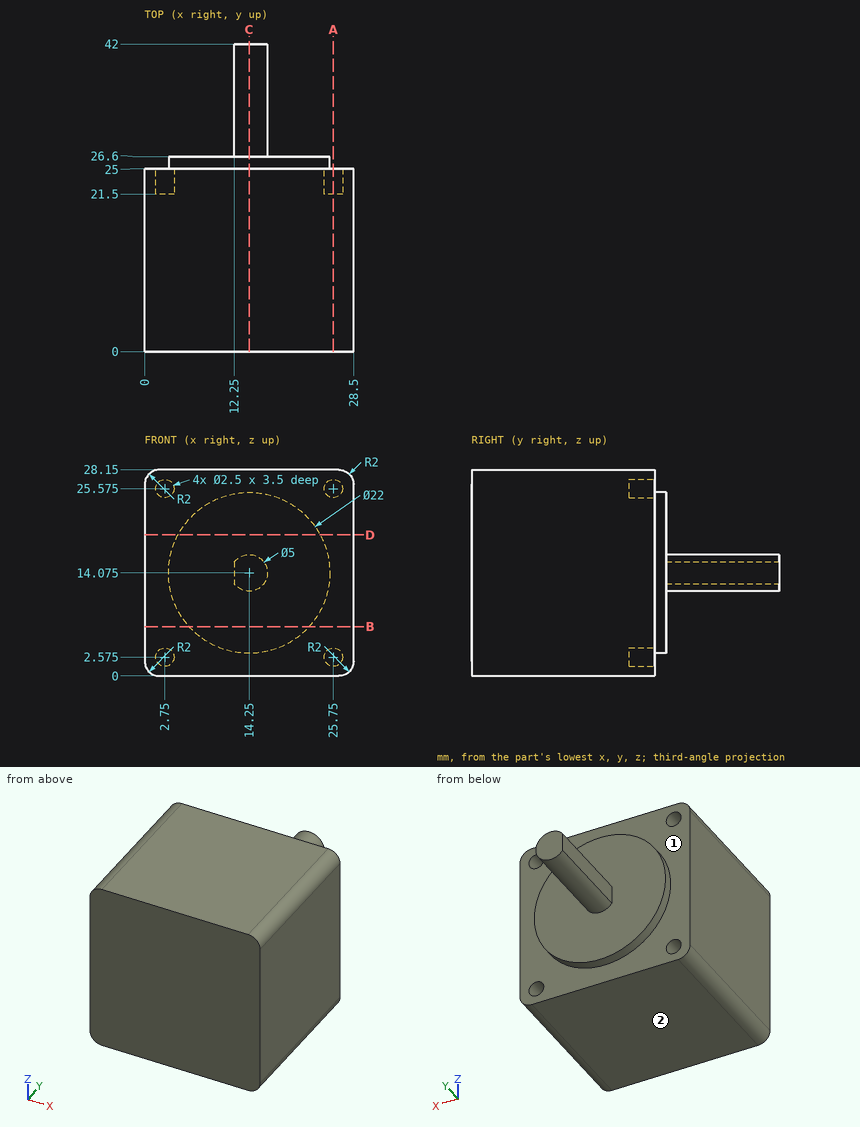
Could you check a few things on this drawing? It's one solid part, dimensions in mm from its lowest x, y, z. A direction names the side the tool comes from. Round coordinates to 2 decimals unless told otherwise and drop trailing zeros. Write each loop counter-clockwise with the first axis right and the second up, starting at its lowest first coordinate (ties: lowest second). Pieces come first, ordered by that corner, then holes. Notation, with made-up numbers: (36, 14.5) -> (93, 14.5) arc R23 ccw to (93, 25.5) -> close; hole circle Ø8 at (-29.75, -28). An arc over 180 degrees is marked (long way). Use one line per item in the form item = value. Start each with the question number.
Q1. Imagine slicing it at B-B (z = 6.75). Please give me the cut outline in (x, y).
Q2. I'm going to push flat-ended pins straight in: P1, Ø1, axis at y = 31, z = 10, coming from the +X side; P2, Ø10, axis at x = 9.5, z = 20, coming from the +Y side; P3, Ø3, axis at x = 2.5, z = 2.5, coming from the +Y side; P4, Ø0.9, axis at y = 35, z = 14.5, coming from the -X side. Where does each tip first touch, or does it pass through?
Q3. Imagine slicing it at A-A (x = 25.75). Please give me the cut outline in (y, z) (3 decimals), then the cut area to 3 significant figures.
Q4. If I drill on probe 1 along Z at (x, y) = (2.75, 23.1) (3 decimals); probe 2 along Y at (x, z) = (26, 2.5); probe 3 along Y at (x, z) = (15.25, 7.5), over which ranges is the centre line in solid material (lowest first)? Write a range as [from, to].
Q5. Imagine slicing it at D-D (z = 19.25). Please give me the cut outline in (x, y).
Q6. Which directions (+Z, -Z, +X, -X, +Y, -Y) give clear straight access to the entire face, cutting with the end or side of a thin tool? Please do the marked faces 1 and 2.
Q7. Imagine slicing it at C-C (x = 14.25). Please give me the cut outline in (y, z) (3 decimals).
Worked out:
q1.outline = (0, 0) -> (28.5, 0) -> (28.5, 25) -> (22.46, 25) -> (22.46, 26.6) -> (6.04, 26.6) -> (6.04, 25) -> (0, 25) -> close
q2.P1 = through
q2.P2 = 26.6
q2.P3 = 25
q2.P4 = 12.25
q3.outline = (0, 0) -> (25, 0) -> (25, 1.325) -> (21.5, 1.325) -> (21.5, 3.825) -> (25, 3.825) -> (25, 24.325) -> (21.5, 24.325) -> (21.5, 26.825) -> (25, 26.825) -> (25, 28.15) -> (0, 28.15) -> close
q3.area = 686 mm^2
q4.probe_1 = [0, 1.325], [3.825, 24.325], [26.825, 28.15]
q4.probe_2 = [0, 21.5]
q4.probe_3 = [0, 26.6]
q5.outline = (0, 0) -> (28.5, 0) -> (28.5, 25) -> (23.96, 25) -> (23.96, 26.6) -> (4.54, 26.6) -> (4.54, 25) -> (0, 25) -> close
q6.face_1 = +Y
q6.face_2 = -Z, +X, -X, +Y, -Y
q7.outline = (0, 0) -> (25, 0) -> (25, 3.075) -> (26.6, 3.075) -> (26.6, 11.575) -> (42, 11.575) -> (42, 16.575) -> (26.6, 16.575) -> (26.6, 25.075) -> (25, 25.075) -> (25, 28.15) -> (0, 28.15) -> close
